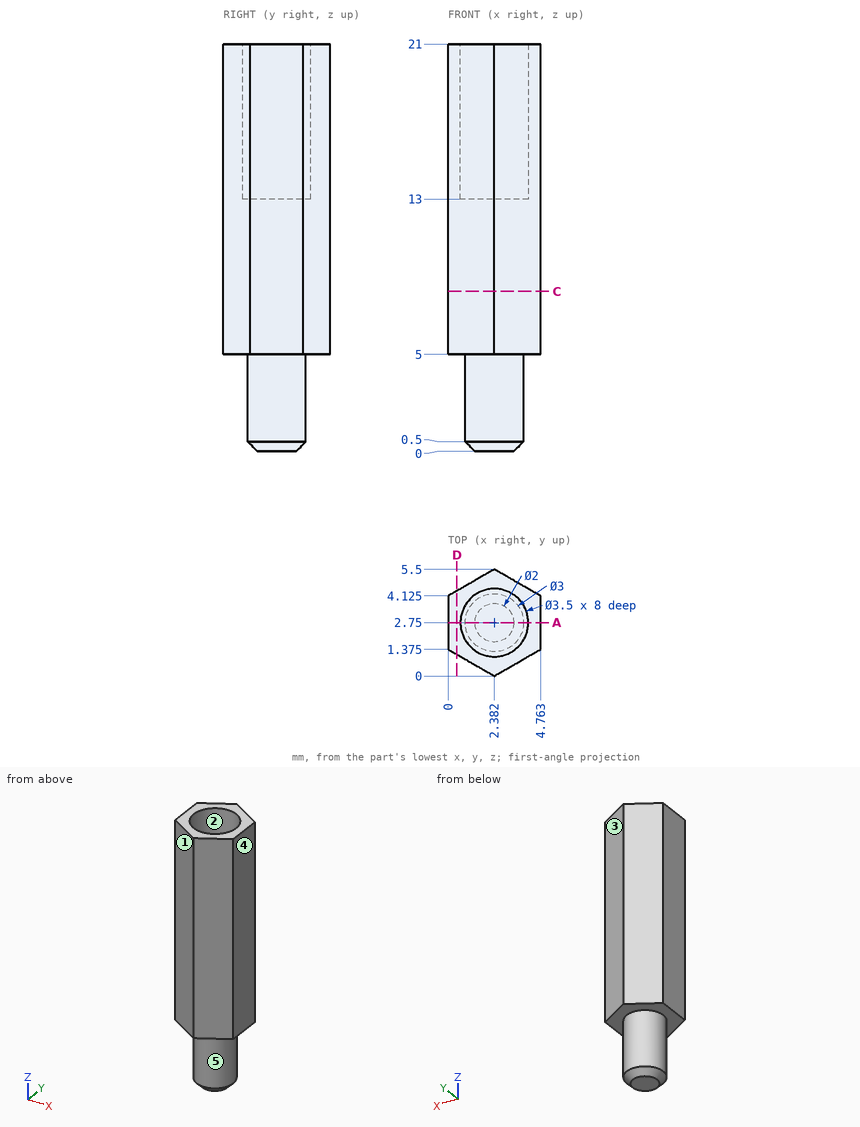
Here's the drawing with two shaded views (mm, measured from the low corner). I have some questions. A direction names the side the tool comes from. Coordinates: 2 decimals unless noted, no trailing zeros. Loops run counter-clockwise (first coordinate to the right, second up) from the corner with the lowest first, then second, coordinate; pieces in that order, holes last. Notation, with made-up numbers: M 52,37 L 74,37 A24 ccw 74,53 Z; hole C 43.5,4 d1. An arc over 180 degrees is marked long. Put each result on its own line as item: value. Start each with the question number.
(1) Imagine slicing it at C-C on z = 8.25. List the corners of the cut face in (x, y) for me (1 decimal).
(2) Imagine slicing it at A-A on y = 2.75. List the corners of the cut face in (x, z) for me.
(3) We'd pull the mould along X, two halves only. Please class the marked faces 1, 2 and 3: +X half, -X half, draft (parallel to the pull), parting line (faces both ways), or undercut.
(4) Which directions (+Z, -Z, +X, -X, +Y, -Y) give clear straight access to the entire face, cutting with the end or side of a thin tool? Please do the marked faces 4 and 5.
(5) Imagine slicing it at D-D on x = 0.45. List the corners of the cut face in (y, z) for me (1 decimal).
(6) Will this pin go through, and if not, where does the flat tip stop? pin 1 Ø2 at (x, z) = (3, 9) entering from +Y.
(7) I need wall thicknesses on probe 1 along X at (y, z) = (1.9, 13.75); probe 2 along Z at (x, y) = (4.25, 2.5); probe 3 along Y at (x, z) = (3.5, 4.75). Which ranges of each line are inside material? Lowest first, please.
Worked answers:
1. outline: M 0,1.4 L 2.4,0 L 4.8,1.4 L 4.8,4.1 L 2.4,5.5 L 0,4.1 Z
2. outline: M 0,5 L 0.88,5 L 0.88,0.5 L 1.38,0 L 3.38,0 L 3.88,0.5 L 3.88,5 L 4.76,5 L 4.76,21 L 4.13,21 L 4.13,13 L 0.63,13 L 0.63,21 L 0,21 Z
3. face 1: -X half
3. face 2: undercut
3. face 3: +X half
4. face 4: +Z, -Z, +X, +Y, -Y
4. face 5: -Z
5. outline: M 1.1,5 L 4.4,5 L 4.4,21 L 1.1,21 Z
6. pin 1: stops at y = 5.5
7. probe 1: x = 0 to 0.85, 3.91 to 4.76
7. probe 2: z = 5 to 21
7. probe 3: y = 1.75 to 3.75
